Part print with two shaded views. Sizes in mm from the minimum x, y, z corner. A direction names the side the tool comes from. Round coordinates to 2 decimals unless told otherwise and drop trailing zeros. Order: outer loops, then holes, each group sorted by start corner. A loop starts at its lowest first (then second) coordinate and runs counter-clockwise, first axis right, second up. Notation, with made-up numbers: (66.25, 38) - (115.25, 38) arc R10 ccw to (115.25, 53) - close; hole circle Ø8 at (7, 77.5). An arc over 180 degrees is marked (long way). Use one line per item in the form item = value.
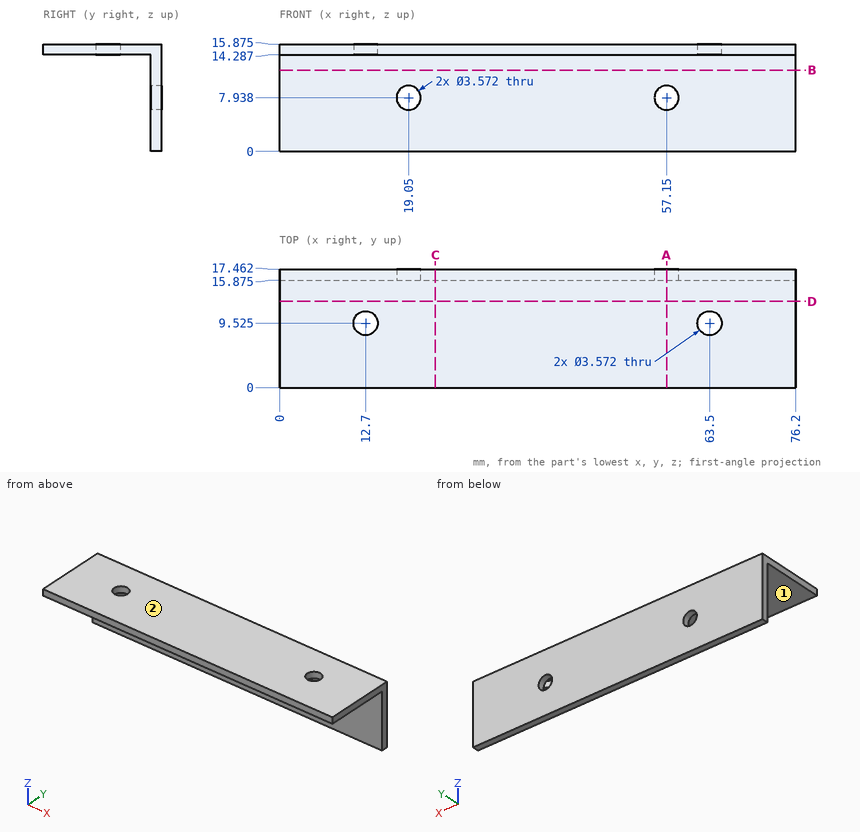
(1) Slice it at D-D on y = 12.75. Give the cut face in (x, z) (1 decimal).
Report:
outline = (0, 14.3) - (76.2, 14.3) - (76.2, 15.9) - (0, 15.9) - close
(2) Probe probe 1 along Y at (x, z) = (12.7, 15.1); probe 2 along Z at (x, y) = (32.5, 6) (1 decimal); probe 3 along Y at (x, z) = (48.5, 8.25) (1 decimal). List the from-to ranges inside material, lowest first. Write a range as [from, to].
Report:
probe_1 = [0, 7.74], [11.31, 17.46]
probe_2 = [14.3, 15.9]
probe_3 = [15.9, 17.5]
(3) Slice it at C-C on x = 23. Give the cut face in (y, z) (1 decimal).
Report:
outline = (0, 14.3) - (15.9, 14.3) - (15.9, 0) - (17.5, 0) - (17.5, 15.9) - (0, 15.9) - close
(4) Tool access for the marked faces 1 and 2: list every direction of +Z, -Z, +X, -X, +Y, -Y with a clear straight run to the whole face (end or side of a thin tool).
Report:
face_1 = -Z, +X, -X, -Y
face_2 = +Z, +X, -X, +Y, -Y
(5) Slice it at A-A on x = 57.15. Give the cut face in (y, z) (1 decimal).
Report:
outline = (0, 14.3) - (15.9, 14.3) - (15.9, 9.7) - (17.5, 9.7) - (17.5, 15.9) - (0, 15.9) - close; (15.9, 0) - (17.5, 0) - (17.5, 6.2) - (15.9, 6.2) - close
(6) Slice it at B-B on z = 12. Give the cut face in (x, y) (1 decimal), then the cut area to 3 significant figures.
Report:
outline = (0, 15.9) - (76.2, 15.9) - (76.2, 17.5) - (0, 17.5) - close
area = 121 mm2
(7) Pin check, flat tips, straight feed: pin 1 (2 mm diameter, centred on x = 44, z = 6, fed in from -Y) (1 decimal); pin 2 (5.5 mm diameter, centred on x = 63.5, y = 9.525, fed in from -Z); pin 3 (4 mm diameter, centred on y = 15.5, z = 4.5, fed in from +X). Stop position of each tip, or through.
Report:
pin_1 = 15.9
pin_2 = 14.29
pin_3 = 76.2
